Build history of the part. All positions in model axes, mm. A direction names the side the tool comes from. Give positions to 0.01 mm unless a question says otherwise; leave off trailing zeros. Order: outer loops, then holes, each group sorted by start corner. A loop starts at its lowest first (then second) coordinate and runs counter-clockwise, first axis right, second up. Notation, with made-up numbers: (-13, 76) -> (35, 76) arc R16 ccw to (35, 102) -> close; hole circle Ø3 at (49, 78.25). An arc over 180 degrees is marked (long way). One line per question, with ' | ' between items. Start each with the question number.
(1) Pull direction Z, two halves, no side cores. Call faces 1 (the face through (1.344, 2.465, 2.284)), 2 (the face through (1.306, 2.465, -2.306)), 3 (the face through (-1, 5, 3)): +Z half, -Z half, draft (parallel to the pull), parting line (faces both ways), or undercut.
(2) Cut at A-A (z = 0). Give the cut face in (x, y) (3 decimals), then the cut area to 3 significant figures.
(3) Pin check, flat tips, straight feed: pin 1 Ø3 at (x, y) = (-3, 1.5) entering from -Z; pin 2 Ø0.9 at (y, z) = (1.5, 0) entering from -X; pin 3 Ø1.5 at (y, z) = (4, 0.5) entering from -X; pin 4 Ø0.9 at (y, z) = (3, 0) entering from +X. Stop position of each tip, or through.
(4) Cut at C-C (y = 2.8). Give the cut face in (x, z), then the cut area to 3 significant figures.
(5) Drill centre lines: L1, parallel to X at y = 1.65, z = -2.25; L2, parallel to X at y = 1.95, z = 3; L3, parallel to Z at x = 1.25, y = 2.1. Where is each one in solid material? Low to high. Write a range as from..to.
(6) Cut at B-B (y = 3.5). Give the cut face in (x, z), then the cut area to 3 significant figures.
(7) Which spindle directions (+Z, -Z, +X, -X, +Y, -Y) get a long thin tool onto all of the face, cutting with end or side? Do faces 4 (the face through (-2.65, 2, 0)), 5 (the face through (-1, 0, 3)). Say none if no direction does.
Autodesk Inventor part; units mm, degrees
ref_plane "Work Plane1" through (0, 2.5, 0) normal (0, 1, 0) x (1, 0, 0)
ref_plane "YZ Plane" through (0, 0, 0) normal (1, 0, 0) x (0, 1, 0)
ref_plane "XZ Plane" through (0, 0, 0) normal (0, 1, 0) x (-1, 0, 0)
sketch "Sketch1" plane through (0, 0, 0) normal (0, 1, 0) x (-1, 0, 0)
  line L0 (2.65, -1.53) -> (0, -3.06)
  line L1 (0, -3.06) -> (-2.65, -1.53)
  line L2 (-2.65, -1.53) -> (-2.65, 1.53)
  line L3 (-2.65, 1.53) -> (0, 3.06)
  line L4 (0, 3.06) -> (2.65, 1.53)
  line L5 (2.65, 1.53) -> (2.65, -1.53)
  circle A0 centre (0, 0) radius 3.5
  dimension "d1" = 5.3
  dimension "d2" = 7
extrude "Extrusion1" add sketch "Sketch1" along normal blind 5
sketch "Sketch2" plane through (0, 0, 0) normal (1, 0, 0) x (0, 1, 0)
  line L0 (0, -3.5) -> (5, -3.5)
  circle A0 centre (2.5, -5.75) radius 2.325
  line L1 (5, -3.5) -> (5, 3.5)
  line L2 (5, -3.5) -> (5, -4.25)
  line L3 (5, -4.25) -> (4.2764, -4.25)
  line L4 (0, -3.5) -> (0, 3.5)
  line L5 (0, -3.5) -> (0, -4.25)
  line L6 (0, -4.25) -> (0.7236, -4.25)
  line L7 (-1, 0) -> (6, 0)
  point P0 (0, 0)
  point P1 (1.9142, -3.5)
  point P2 (3.0858, -3.5)
  dimension "d5" = 4.65
  dimension "d6" = 2.25
  dimension "d7" = 0.75
  dimension "d8" = 0.75
revolve "Revolution1" cut sketch "Sketch2" angle 360 about axis through (0, -10, 0) along (0, 1, 0) contours A0 L0 | L0 A0
revolve "Revolution2" add sketch "Sketch2" angle 360 about axis through (0, -10, 0) along (0, 1, 0) contours L0 A0 L6 L5 | L0 L2 L3 A0
chamfer "Chamfer1" distance 0.5 angle 45 2 edges at (0, 5, 4.25) (0, 0, 4.25)
ref_plane "Work Plane1" through (0, 2.5, 0) normal (0, 1, 0) x (1, 0, 0)
sketch "Sketch3" plane through (0, 0, 0) normal (0, -1, 0) x (1, 0, 0)
  line L0 (-2.65, -1.53) -> (0, -3.06)
  line L1 (-2.65, 1.53) -> (-2.65, -1.53)
  line L2 (0, 3.06) -> (-2.65, 1.53)
  line L3 (2.65, 1.53) -> (0, 3.06)
  line L4 (2.65, -1.53) -> (2.65, 1.53)
  line L5 (0, -3.06) -> (2.65, -1.53)
  circle A0 centre (0, 0) radius 3.75
properties part number "5mm Hex Bearing Inside_3DPrint"
Result set:
1) face 1: undercut | face 2: undercut | face 3: draft
2) outline: (-4.25, 0.5) -> (-3.75, 0) -> (-2.65, 0) -> (-2.65, 5) -> (-3.75, 5) -> (-4.25, 4.5) -> (-4.25, 4.276) arc R2.325 cw to (-4.25, 0.724) -> close; (2.65, 0) -> (3.75, 0) -> (4.25, 0.5) -> (4.25, 0.724) arc R2.325 cw to (4.25, 4.276) -> (4.25, 4.5) -> (3.75, 5) -> (2.65, 5) -> close | area: 11.4 mm2
3) pin 1: stops at z = -3.89 | pin 2: stops at x = -3.93 | pin 3: stops at x = -4.25 | pin 4: stops at x = 3.63
4) outline: circle Ø6.89 at (0, 0); hole (-2.65, -1.53) -> (0, -3.06) -> (2.65, -1.53) -> (2.65, 1.53) -> (0, 3.06) -> (-2.65, 1.53) -> close | area: 12.9 mm2
5) L1: x = -2.79..-1.4, 1.4..2.79 | L2: x = -1.79..-0.1, 0.1..1.79 | L3: z = -3.23..-2.34, 2.34..3.23
6) outline: circle Ø7.3 at (0, 0); hole (-2.65, -1.53) -> (0, -3.06) -> (2.65, -1.53) -> (2.65, 1.53) -> (0, 3.06) -> (-2.65, 1.53) -> close | area: 17.6 mm2
7) face 4: +Y, -Y | face 5: +Z, -Z, +X, -X, -Y
